```python
from build123d import *

# Parameters (mm, degrees)
F0_R     = 37.5
F1_DEPTH = 19
F2_T     = -2.5
F3_R     = 3.75
F4_DEPTH = 19.001
F6_DEPTH = 4
F8_DEPTH = 4


with BuildPart() as f1:
    # F0 (on Front) → F1 (new body)
    with BuildSketch(Plane.XZ):
        Circle(F0_R)
    extrude(amount=F1_DEPTH)

    # F2
    f2_openings = [f1.faces().sort_by_distance(p)[0] for p in [
        (0, 0, 0),
    ]]
    offset(amount=F2_T, openings=f2_openings)

    # F3 (on face) → F4 (cut, through all)
    with BuildSketch(Plane.XZ.offset(19)):
        Circle(F3_R)
    extrude(amount=-F4_DEPTH, mode=Mode.SUBTRACT)

    # F5 (on face) → F6 (join)
    with BuildSketch(Plane(origin=(0, 0, 0), x_dir=(-1, 0, 0), z_dir=(0, 1, 0))):
        with BuildLine():
            ThreePointArc((21.3985376308, 27.696616892), (0, 35), (-21.3985376308, 27.696616892))
            Line((-21.3985376308, 27.696616892), (21.3985376308, 27.696616892))
        make_face()
    extrude(amount=-F6_DEPTH)

    # F7 (on face) → F8 (join)
    with BuildSketch(Plane(origin=(0, 0, 0), x_dir=(-1, 0, 0), z_dir=(0, 1, 0))):
        with BuildLine():
            Line((21.3985376308, -27.696616892), (-21.3985376308, -27.696616892))
            ThreePointArc((-21.3985376308, -27.696616892), (0, -35), (21.3985376308, -27.696616892))
        make_face()
    extrude(amount=-F8_DEPTH)


solid = f1.part
```
CAD build for the part. Positions are in the model's coordinates, mm. A direction names the side the tool comes from. Coordinates: 2 decimals unless noted, no trailing zeros. Write each loop counter-clockwise with the first axis right and the second up, starting at its lowest first coordinate (ties: lowest second). Pieces come first, ordered by that corner, then holes. Notation, with made-up numbers: (56, 89.5) -> (97, 89.5) arc R22 ccw to (97, 102.5) -> close; hole circle Ø8 at (15, -5.75). An arc over 180 degrees is marked (long way). Return JSON: item names as keys, results as strings. Group by question number.
Q1. Drill centre lines: line 1 (Z direction, x = 0, y = -17.15); line 2 (Y direction, x = -4.5, z = 28.5); line 3 (Y direction, x = -6, z = -2). Where is each one in solid material? Low to high.
Q2. Cut at B-B, the plane z = 0. Give the cut face in (x, y).
Q3. Cut at C-C, the plane y = -14.25. Give the cut face in (x, z), then the cut area to 3 significant figures.
Q4. Flat gauge pins, fed straight in: pin 1 (5 mm diameter, centred on x = 3.5, y = -7.5, fed in from -Z); pin 2 (3 mm diameter, centred on x = -8.5, y = -2, fed in from -Z); pin 3 (8 mm diameter, centred on y = -10.5, z = 19.5, fed in from +X). Where does each tip first touch, or does it go through?
Q5. Cut at D-D, the plane z = 26.5. Give the cut face in (x, y).
Q6. Pull direction Y, two halves, no side cores. Call faces 4 (the face through (-3.746, -17.768, 0.165)), 5 (the face through (-34.966, -8.134, 1.539)), 6 (the face through (8, -19, 1)): released by +Y, released by -Y, zero draft, split by the parting line, or undercut.
Q7. Which spindle directions (+Z, -Z, +X, -X, +Y, -Y) get a long thin tool onto all of the face, cutting with end or side? Do faces 1 (the face through (0, -2, 27.697)), 2 (the face through (0, -4, 31)), 3 (the face through (0, 0, 28)). Say none if no direction does.
Q8. Cut at A-A, the plane x = 0. Give the cut face in (y, z), then the cut area to 3 significant figures.
Returned:
{
 "1": {"line 1": "z = -37.5 to -3.75, 3.75 to 37.5", "line 2": "y = -19 to -16.5, -4 to 0", "line 3": "y = -19 to -16.5"},
 "2": {"outline": "(-37.5, -19) -> (-3.75, -19) -> (-3.75, -16.5) -> (-35, -16.5) -> (-35, 0) -> (-37.5, 0) -> close; (3.75, -19) -> (37.5, -19) -> (37.5, 0) -> (35, 0) -> (35, -16.5) -> (3.75, -16.5) -> close"},
 "3": {"outline": "circle Ø75 at (0, 0); hole circle Ø70 at (0, 0)", "area": "569 mm2"},
 "4": {"pin 1": "stops at z = -37.49", "pin 2": "stops at z = -36.84", "pin 3": "stops at x = 34.15"},
 "5": {"outline": "(-26.53, -19) -> (26.53, -19) -> (26.53, 0) -> (22.86, 0) -> (22.86, -16.5) -> (-22.86, -16.5) -> (-22.86, 0) -> (-26.53, 0) -> close"},
 "6": {"face 4": "zero draft", "face 5": "undercut", "face 6": "released by -Y"},
 "7": {"face 1": "+Y", "face 2": "none", "face 3": "+Z, -Z, +X, -X, +Y"},
 "8": {"outline": "(-19, -37.5) -> (0, -37.5) -> (0, -27.7) -> (-4, -27.7) -> (-4, -35) -> (-16.5, -35) -> (-16.5, -3.75) -> (-19, -3.75) -> close; (-19, 3.75) -> (-16.5, 3.75) -> (-16.5, 35) -> (-4, 35) -> (-4, 27.7) -> (0, 27.7) -> (0, 37.5) -> (-19, 37.5) -> close", "area": "310 mm2"}
}
